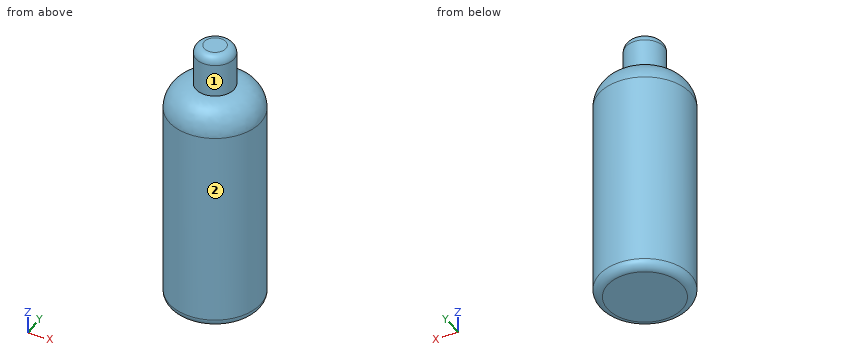
```python
from build123d import *

# Parameters (mm, degrees)
F2_R     = 11.5
F3_DEPTH = 25
F4_R     = 5
F5_R     = 5


with BuildPart() as f1:
    # F0 (on Front) → F1 (revolve)
    with BuildSketch(Plane.XZ):
        with BuildLine():
            Line((0, 140), (0, 0))
            Line((0, 0), (27.5, 0))
            Line((27.5, 0), (27.5, 124))
            ThreePointArc((27.5, 124), (22.813708, 135.313708), (11.5, 140))
            Line((11.5, 140), (0, 140))
        make_face()
    revolve(axis=Axis((0, 0, 70), (0, 0, -1)))

    # F2 (on face) → F3 (join)
    with BuildSketch(Plane.XY.offset(140)):
        Circle(F2_R)
    extrude(amount=F3_DEPTH)

    # F4
    f4_edges = [f1.edges().sort_by_distance(p)[0] for p in [
        (-11.5, 0, 165),
    ]]
    fillet(f4_edges, radius=F4_R)

    # F5
    f5_edges = [f1.edges().sort_by_distance(p)[0] for p in [
        (-27.5, 0, 0),
    ]]
    fillet(f5_edges, radius=F5_R)


solid = f1.part
```
Geometry check sheet. Reference: the model listing, model coordinates, mm. Face numbers are marked on the shaded views. A direction names the side the tool comes from. Round coordinates to 2 decimals unless told otherwise and drop trailing zeros. Loops run counter-clockwise (first coordinate to the right, second up) from the corner with the lowest first, then second, coordinate; pieces in that order, holes last. Notation, with made-up numbers: (56.25, 38) - (104.25, 38) arc R17 ccw to (104.25, 63) - close; hole circle Ø9 at (11, -13). An arc over 180 degrees is marked (long way). Use a Markdown table: item, result.
Q1. Cross-section at A-A on z = 106. Record the cut outline in (x, y), plus the area to 3 significant figures.
Solutions:
| item | result |
|---|---|
| outline | circle Ø55 at (0, 0) |
| area | 2,380 mm2 |
Q2. Access from +Z, -Z, +X, -X, +Y, -Y to the whole of each face (thin tool, end or side, straight path). Record for the marked faces 1 and 2.
Solutions:
| item | result |
|---|---|
| face 1 | +Z |
| face 2 | +Z, -Z |
Q3. Material ranges on line 1 (Z direction, x = 5.5, y = -4); line 2 (Z direction, x = -12, y = 1.5); line 3 (Y direction, x = -18, z = 36), recorded low to high.
Solutions:
| item | result |
|---|---|
| line 1 | z = 0 to 164.99 |
| line 2 | z = 0 to 139.99 |
| line 3 | y = -20.79 to 20.79 |
Q4. Go/stop test with flat-tipped pins: P1, Ø4, axis at x = 15.5, z = 47, coming from the -Y side; P2, Ø1.5, axis at y = 2.5, z = 121, coming from the -X side; P3, Ø1, axis at x = 4.5, y = -18.5, coming from the -Z side; P4, Ø5, axis at y = -21, z = 73, coming from the -X side. Record where each tip stops, or that it passes through.
Solutions:
| item | result |
|---|---|
| P1 | stops at y = -23.96 |
| P2 | stops at x = -27.44 |
| P3 | stops at z = 0 |
| P4 | stops at x = -20.35 |
